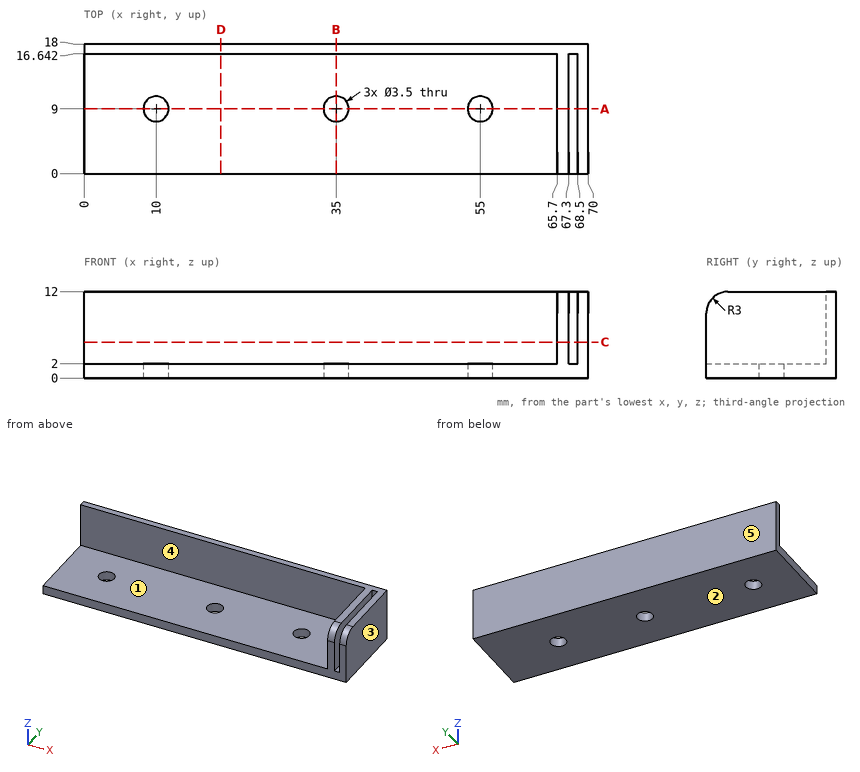
Geometry check sheet. Reference: drawing and pictorial views, mm from the part's lowest x, y, z. A direction names the side the tool comes from. Coordinates: 2 decimals unless noted, no trailing zeros. Order: outer loops, then holes, each group sorted by start corner. A loop starts at its lowest first (then second) coordinate and runs counter-clockwise, first axis right, second up. Notation, with made-up numbers: (48.5, 25.5) -> (64.5, 25.5) arc R37 ccw to (64.5, 63.5) -> close; hole circle Ø1 at (66.25, 88.25). An arc over 180 degrees is marked (long way). Put each result on its own line as item: value. Start each with the question number.
1) Cross-section at D-D (x = 19). Enter the section's corners in (y, z).
2) Material ranges on L1, parallel to Y at x = 35, z = 0.6; L2, parallel to X at y = 15.25, z = 10.25; L3, parallel to X at y = 10.25, z = 1.5 (1 decimal), recorded low to high.
3) Release check for a two-part mould opening along Y. For the marked faces 3, 4 and 5 record: pulls with the +Y half, pulls with the -Y half, needs draft (parallel to the pull), parting line crosses it, or undercut.
4) Tool access check on the marked faces 1 and 2. Record the directions out of +Z, -Z, +X, -X, +Y, -Y that give a thin tool (end or side, any length) a straight path to the whole face; none if there is none.
5) Cross-section at A-A (y = 9). Enter the section's corners in (x, z), plus the area to 3 significant figures.
6) Go/stop test with flat-tipped pins: pin 1 (1.5 mm diameter, centred on x = 10, y = 13, fed in from +Z); pin 2 (0.6 mm diameter, centred on x = 68, z = 5, fed in from -Y). Record where each tip stops, or that it passes through.
7) Cross-section at C-C (z = 5). Enter the section's corners in (x, y).
8) Cross-section at B-B (x = 35). Enter the section's corners in (y, z).
Geometry check:
1. outline: (0, 0) -> (18, 0) -> (18, 12) -> (16.64, 12) -> (16.64, 2) -> (0, 2) -> close
2. L1: y = 0 to 7.25, 10.75 to 18
2. L2: x = 65.7 to 67.3, 68.5 to 70
2. L3: x = 0 to 8.8, 11.2 to 33.8, 36.2 to 53.8, 56.2 to 70
3. face 3: needs draft
3. face 4: pulls with the -Y half
3. face 5: pulls with the +Y half
4. face 1: +Z, -X, -Y
4. face 2: -Z, +X, -X, +Y, -Y
5. outline: (0, 0) -> (8.25, 0) -> (8.25, 2) -> (0, 2) -> close; (11.75, 0) -> (33.25, 0) -> (33.25, 2) -> (11.75, 2) -> close; (36.75, 0) -> (53.25, 0) -> (53.25, 2) -> (36.75, 2) -> close; (56.75, 0) -> (70, 0) -> (70, 12) -> (68.5, 12) -> (68.5, 2) -> (67.3, 2) -> (67.3, 12) -> (65.7, 12) -> (65.7, 2) -> (56.75, 2) -> close
5. area: 150 mm^2
6. pin 1: stops at z = 2
6. pin 2: stops at y = 16.64
7. outline: (0, 16.64) -> (65.7, 16.64) -> (65.7, 0) -> (67.3, 0) -> (67.3, 16.64) -> (68.5, 16.64) -> (68.5, 0) -> (70, 0) -> (70, 18) -> (0, 18) -> close
8. outline: (0, 0) -> (7.25, 0) -> (7.25, 2) -> (0, 2) -> close; (10.75, 0) -> (18, 0) -> (18, 12) -> (16.64, 12) -> (16.64, 2) -> (10.75, 2) -> close
